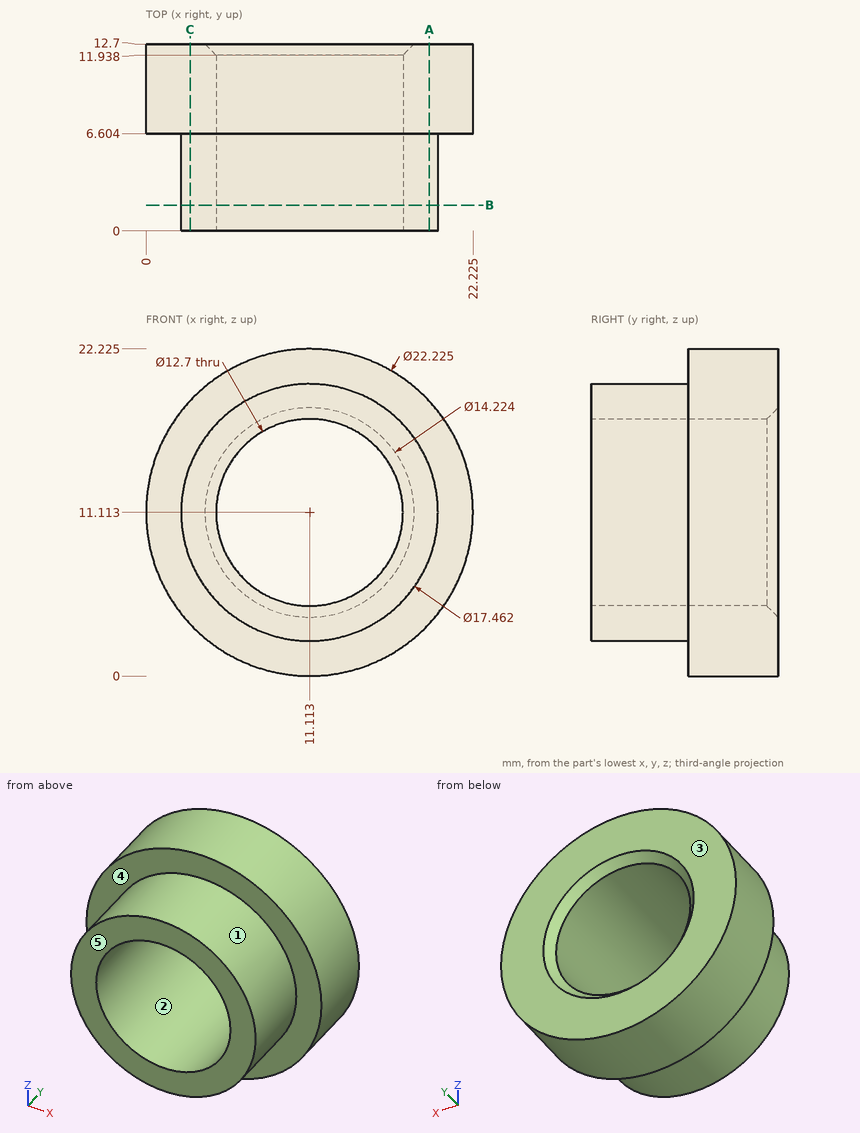
Part print with two shaded views. Sizes in mm from the minimum x, y, z corner. A direction names the side the tool comes from. Give positions to 0.01 mm unless a question says otherwise; leave off trailing zeros. Loops run counter-clockwise (first coordinate to the right, second up) from the corner with the lowest first, then second, coordinate; pieces in that order, holes last. Notation, with made-up numbers: (8.5, 63) - (32.5, 63) arc R15 ccw to (32.5, 92) - close; hole circle Ø8 at (-28, 75.5). An arc over 180 degrees is marked (long way). Put each result on its own line as item: value.
Q1. Slice it at B-B (y = 1.75). Give the cut face in (x, z).
Filled in:
outline: circle Ø17.46 at (11.11, 11.11); hole circle Ø12.7 at (11.11, 11.11)
Q2. Mould opens along X. For the marked faces 1, 2 and 3 say: pulls with the +X half, pulls with the -X half, needs draft (parallel to the pull), parting line crosses it, or undercut.
Filled in:
face 1: parting line crosses it
face 2: undercut
face 3: needs draft
Q3. Slice it at A-A (x = 19.25). Give the cut face in (y, z) (1 decimal), plus the area to 3 significant figures.
Filled in:
outline: (0, 7.9) - (6.6, 7.9) - (6.6, 3.5) - (12.7, 3.5) - (12.7, 18.7) - (6.6, 18.7) - (6.6, 14.3) - (0, 14.3) - close
area: 134 mm²
Q4. Probe line 1 along X through (y, z) = (1.25, 11); line 2 along X through (y, z) = (9.5, 11) (1 decimal); line 3 along Z through (x, y) = (11.25, 2.25) (1 decimal). List the from-to ranges inside material, lowest first.
Filled in:
line 1: x = 2.38 to 4.76, 17.46 to 19.84
line 2: x = 0 to 4.8, 17.5 to 22.2
line 3: z = 2.4 to 4.8, 17.5 to 19.8
Q5. Tool access for the marked faces 4 and 5: list every direction of +Z, -Z, +X, -X, +Y, -Y with a clear straight run to the whole face (end or side of a thin tool).
Filled in:
face 4: -Y
face 5: +Z, -Z, +X, -X, -Y
Q6. Flat gauge pins, fed straight in: pin 1 (3 mm diameter, centred on x = 15.5, y = 6.5, fed in from -Z); pin 2 (1.5 mm diameter, centred on x = 4.5, y = 11, fed in from -Z); pin 3 (6 mm diameter, centred on x = 4.5, y = 9, fed in from -Z). Where does each tip first touch, or does it go through?
Filled in:
pin 1: stops at z = 0.38
pin 2: stops at z = 1.67
pin 3: stops at z = 0.6
